from build123d import *

# Parameters (mm, degrees)
SALIENTE_EXTRUIR1_DEPTH = 18
CORTAR_EXTRUIR1_DEPTH   = 14
CROQUIS3_W              = 40
CROQUIS3_H              = 16
SALIENTE_EXTRUIR2_DEPTH = 2
CROQUIS10_R             = 1.5
CORTAR_EXTRUIR2_DEPTH   = 10


with BuildPart() as part:
    # Croquis1 → Saliente-Extruir1 (new body)
    with BuildSketch(Plane.XY):
        Polygon((-49.27736704, 8.428571429), (-49.27736704, -14.571428571), (-9.27736704, -14.571428571), (-9.27736704, 8.428571429), (-16.27736704, 8.428571429), (-16.27736704, 18.428571429), (-44.27736704, 18.428571429), (-44.27736704, 8.428571429), align=None)
    extrude(amount=SALIENTE_EXTRUIR1_DEPTH)

    # Croquis2 → Cortar-Extruir1 (cut)
    with BuildSketch(Plane.XY.offset(18)):
        Polygon((-9.27736704, 6.428571429), (-9.27736704, -9.571428571), (-49.27736704, -9.571428571), (-49.27736704, 6.428571429), (-41.27736704, 6.428571429), (-41.27736704, 18.428571429), (-19.27736704, 18.428571429), (-19.27736704, 6.428571429), align=None)
    extrude(amount=-CORTAR_EXTRUIR1_DEPTH, mode=Mode.SUBTRACT)

    # Croquis3 → Saliente-Extruir2 (add)
    with BuildSketch(Plane.XY.offset(4)):
        with Locations((-29.27736704, -1.571428571)):
            Rectangle(CROQUIS3_W, CROQUIS3_H)
    extrude(amount=SALIENTE_EXTRUIR2_DEPTH)

    # Croquis10 → Cortar-Extruir2 (cut)
    with BuildSketch(Plane.XY.offset(18)):
        with Locations((-46.77736704, -12.071428571)):
            Circle(CROQUIS10_R)
        with Locations((-11.77736704, -12.071428571)):
            Circle(CROQUIS10_R)
    extrude(amount=-CORTAR_EXTRUIR2_DEPTH, mode=Mode.SUBTRACT)


solid = part.part
Verification items for the finished model (mm, model axes). A direction names the side the tool comes from. Give positions to 0.01 mm unless a question says otherwise; leave off trailing zeros. Loops run counter-clockwise (first coordinate to the right, second up) from the corner with the lowest first, then second, coordinate; pieces in that order, holes last.
1) Sectioned sample at D-D, the plane z = 11.5. Enter the section's corners in (x, y).
2) Thickness scan on line 1 along X through (y, z) = (7.5, 16.5); line 2 along Y through (x, z) = (-46, 13.75); line 3 along X through (y, z) = (13, 11.75). Record the ranges inside material, lowest first.
3) Set-up check for faces 1 (the flat face through (-16.277, 13, 9)), 2 (the flat face through (-44.277, 13, 9)), 3 (the flat face through (-14, 6.429, 12)): record each of +Z, -Z, +X, -X, +Y, -Y from which the full face is reachable in a straight line by a thin tool's end or side.
4) Sectioned sample at B-B, the plane z = 1.25. Enter the section's corners in (x, y).
5) Sectioned sample at C-C, the plane x = -18. Enter the section's corners in (y, z), then the cut area to 3 significant figures.
6) Draft check along Y on faces 4 (the flat face through (-13, 8.429, 9)), 5 (the flat face through (-9.277, -3, 5)), 6 (the flat face through (-29, -9.571, 12)), 7 (the cylindrical face through (-11.085, -13.402, 13.07)). Enter one of: pulls with the +Y half, pulls with the -Y half, needs draft (parallel to the pull), parting line crosses it, or undercut.
7) Depth check by flat-ended pin: pin 1 Ø8 at (y, z) = (14, 11.5) entering from -X; pin 2 Ø3.5 at (x, z) = (-12.5, 9.5) entering from +Y; pin 3 Ø6 at (x, y) = (-43.5, -3.5) entering from +Z. Enter the tip coordinate at first touch or a pass-through.
8) Sectioned sample at A-A, the plane z = 6.75. Enter the section's corners in (x, y), then the cut area to 3 significant figures.
Answers:
1. outline: (-49.28, -14.57) - (-9.28, -14.57) - (-9.28, -9.57) - (-49.28, -9.57) - close; (-49.28, 6.43) - (-41.28, 6.43) - (-41.28, 18.43) - (-44.28, 18.43) - (-44.28, 8.43) - (-49.28, 8.43) - close; (-19.28, 6.43) - (-9.28, 6.43) - (-9.28, 8.43) - (-16.28, 8.43) - (-16.28, 18.43) - (-19.28, 18.43) - close; hole circle Ø3 at (-46.78, -12.07); hole circle Ø3 at (-11.78, -12.07)
2. line 1: x = -49.28 to -41.28, -19.28 to -9.28
2. line 2: y = -14.57 to -13.35, -10.79 to -9.57, 6.43 to 8.43
2. line 3: x = -44.28 to -41.28, -19.28 to -16.28
3. face 1: +Z, -Z, +X, +Y
3. face 2: +Z, -Z, -X, +Y
3. face 3: +Z, +X, -X
4. outline: (-49.28, -14.57) - (-9.28, -14.57) - (-9.28, 8.43) - (-16.28, 8.43) - (-16.28, 18.43) - (-44.28, 18.43) - (-44.28, 8.43) - (-49.28, 8.43) - close
5. outline: (-14.57, 0) - (18.43, 0) - (18.43, 18) - (6.43, 18) - (6.43, 6) - (-9.57, 6) - (-9.57, 18) - (-14.57, 18) - close
5. area: 402 mm2
6. face 4: pulls with the +Y half
6. face 5: needs draft
6. face 6: undercut
6. face 7: undercut
7. pin 1: stops at x = -44.28
7. pin 2: stops at y = 8.43
7. pin 3: stops at z = 6
8. outline: (-49.28, -14.57) - (-9.28, -14.57) - (-9.28, -9.57) - (-49.28, -9.57) - close; (-49.28, 6.43) - (-41.28, 6.43) - (-41.28, 18.43) - (-44.28, 18.43) - (-44.28, 8.43) - (-49.28, 8.43) - close; (-19.28, 6.43) - (-9.28, 6.43) - (-9.28, 8.43) - (-16.28, 8.43) - (-16.28, 18.43) - (-19.28, 18.43) - close
8. area: 296 mm2
